Input: dimensioned drawing with shaded views. Units: mm. Origin: part minimum x, y, z. Give positions to 0.01 mm unless a question says otherwise; leave off trailing zeros. Loops run counter-clockwise (first coordinate to the right, second up) from the corner with the lowest first, then second, coordinate; pieces in that order, holes last. Notation, with made-up numbers: (-5, 88.5) -> (23, 88.5) arc R11 cw to (23, 101.5) -> close; hole circle Ø4 at (74.25, -21). An arc over 180 degrees is marked (long way). Answer in a Markdown table with one row per item. Add a question column.
1) Line query: line 1 (Z direction, x = 19.5, y = 5.3); line 2 (Z direction, x = 45.5, y = 1.75); line 3 (Z direction, x = 5.5, y = 2.4). Output: solid intervals per line, ascending. Write a range as from..to.
2) Section query C-C (z = 31). Return the cut outline in (x, y), plus the area to 3 significant figures.
3) Draft query along X for the marked faces 1, 2 and 3. Return one class per face: +X half, -X half, draft (parallel to the pull), parting line (faces both ways), or undercut.
4) First-contact query: P1, Ø4, axis at x = 19.5, z = 5, coming from the +Y side; P2, Ø4.5, axis at x = 5.5, z = 3, coming from the +Y side; P3, Ø5, axis at x = 45.5, z = 31, coming from the -Y side. Flat tips, straight axial feed; report the tip coordinate or a pass-through.
5) Section query D-D (x = 19.5). Return the cut outline in (y, z).
6) Section query B-B (y = 1). Return the cut outline in (x, z), plus the area to 3 significant figures.
7) Section query A-A (x = 32.5). Return the cut outline in (y, z).
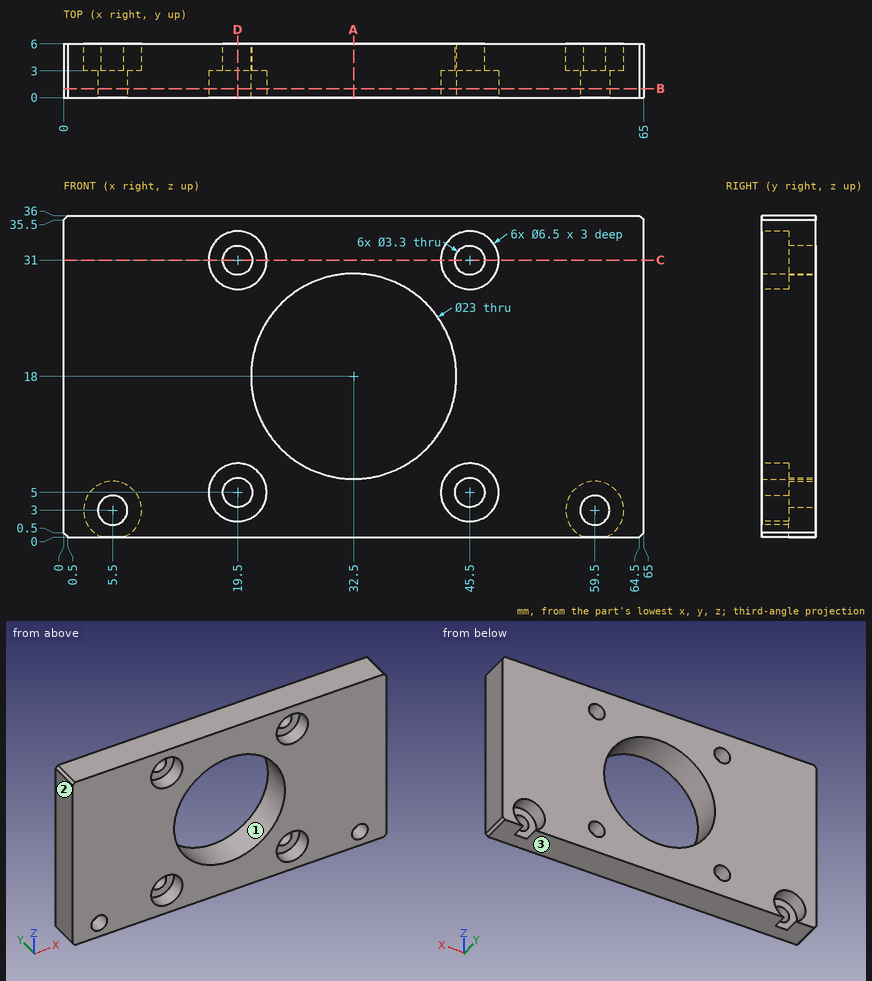
Evaluation:
| question | item | result |
|---|---|---|
| 1 | line 1 | 0..3.35, 6.65..29.35, 32.65..36 |
| 1 | line 2 | 0..1.75, 8.25..27.75, 34.25..36 |
| 1 | line 3 | 0..1.35, 4.65..36 |
| 2 | outline | (0, 0) -> (16.25, 0) -> (16.25, 3) -> (17.85, 3) -> (17.85, 6) -> (0, 6) -> close; (21.15, 3) -> (22.75, 3) -> (22.75, 0) -> (42.25, 0) -> (42.25, 3) -> (43.85, 3) -> (43.85, 6) -> (21.15, 6) -> close; (47.15, 3) -> (48.75, 3) -> (48.75, 0) -> (65, 0) -> (65, 6) -> (47.15, 6) -> close |
| 2 | area | 331 mm² |
| 3 | face 1 | undercut |
| 3 | face 2 | -X half |
| 3 | face 3 | draft |
| 4 | P1 | y = 6 |
| 4 | P2 | y = 3 |
| 4 | P3 | y = 3 |
| 5 | outline | (0, 0) -> (6, 0) -> (6, 3.35) -> (3, 3.35) -> (3, 1.75) -> (0, 1.75) -> close; (0, 8.25) -> (3, 8.25) -> (3, 6.65) -> (6, 6.65) -> (6, 29.35) -> (3, 29.35) -> (3, 27.75) -> (0, 27.75) -> close; (0, 34.25) -> (3, 34.25) -> (3, 32.65) -> (6, 32.65) -> (6, 36) -> (0, 36) -> close |
| 6 | outline | (0, 0.5) -> (0.5, 0) -> (64.5, 0) -> (65, 0.5) -> (65, 35.5) -> (64.5, 36) -> (0.5, 36) -> (0, 35.5) -> close; hole circle Ø3.3 at (5.5, 3); hole circle Ø6.5 at (19.5, 5); hole circle Ø6.5 at (19.5, 31); hole circle Ø23 at (32.5, 18); hole circle Ø6.5 at (45.5, 5); hole circle Ø6.5 at (45.5, 31); hole circle Ø3.3 at (59.5, 3) |
| 6 | area | 1,770 mm² |
| 7 | outline | (0, 0) -> (6, 0) -> (6, 6.5) -> (0, 6.5) -> close; (0, 29.5) -> (6, 29.5) -> (6, 36) -> (0, 36) -> close |
